```python
from build123d import *

# Parameters (mm, degrees)
F1_DEPTH = 10
F2_W     = 5
F2_H     = 5
F3_DEPTH = 5
F4_W     = 5
F4_H     = 5
F5_DEPTH = 2
F6_SIZE  = 1


with BuildPart() as f1:
    # F0 (on Front) → F1 (new body)
    with BuildSketch(Plane.XZ):
        Polygon((0, 49.2), (0, 0), (21.76041, 48.874682), (14.42041, 48.874682), (6.8, 31.7), (6.8, 49.2), align=None)
    extrude(amount=F1_DEPTH)

    # F2 (on face) → F3 (cut)
    with BuildSketch(Plane.XY.offset(49.2)):
        with Locations((3.4, -5)):
            Rectangle(F2_W, F2_H)
    extrude(amount=-F3_DEPTH, mode=Mode.SUBTRACT)

    # F4 (on face) → F5 (cut)
    with BuildSketch(Plane.XY.offset(48.874682)):
        with Locations((18.09041, -5)):
            Rectangle(F4_W, F4_H)
    extrude(amount=-F5_DEPTH, mode=Mode.SUBTRACT)

    # F6
    f6_edges = [f1.edges().sort_by_distance(p)[0] for p in [
        (6.8, -10, 40.45),
        (0, -10, 24.6),
        (10.610205, -10, 40.287341),
        (6.8, 0, 40.45),
        (10.880205, 0, 24.437341),
        (10.610205, 0, 40.287341),
        (10.880205, -10, 24.437341),
        (0, 0, 24.6),
    ]]
    chamfer(f6_edges, length=F6_SIZE)


solid = f1.part
```
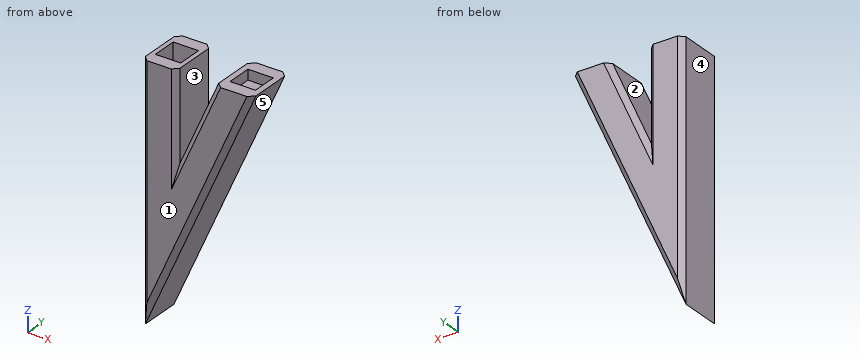
Model file for the job. Use its own axes, mm. Face numbers are marked on the shaded views. A direction names the side the tool comes from. Coordinates: 2 decimals unless noted, no trailing zeros. Write each loop counter-clockwise with the first axis right and the second up, starting at its lowest first coordinate (ties: lowest second). Pieces come first, ordered by that corner, then holes. Notation, with made-up numbers: (-18.5, -18) - (22.5, -18) arc R24 cw to (22.5, -4) - close; hole circle Ø7 at (-3, 33.25). An arc over 180 degrees is marked (long way). Use a Markdown table: item, result. Add a question column.
Item 1: 3-axis set-ups, long thin cutter, end or side, ignore diameter. For the marked faces 1 and 2: which of +Z, -Z, +X, -X, +Y, -Y reach the whole face in a straight line?
Item 2: Band-saw the part on D-D, the plane z = 21.5. Write the cut outline in (x, y).
Item 3: Two-plate mould, pull along X, no slides. Class the marked faces 3, 4 and 5: pulls with the +X half, pulls with the -X half, needs draft (parallel to the pull), parting line crosses it, or undercut.
Item 4: Band-saw the part on B-B, the plane z = 41.5. Write the cut outline in (x, y), and give its area (3 significant figures).
Item 5: Band-saw the part on A-A, the plane y = -4.25. Write the cut outline in (x, z), and give its area (3 significant figures).
Item 6: Drill centre lines: line 1 along X through (y, z) = (-2, 40); line 2 along X through (y, z) = (-9, 37.5); line 3 along Y through (x, z) = (18.75, 44). Where is each one in solid material? Low to high.
Item 7: Band-saw the part on C-C, the plane x = 2.5. Write the cut outline in (y, z), and give its area (3 significant figures).
Item 8: Drop flat-ended pins along their axis: pin 1 (2 mm diameter, centred on y = -1.5, z = 21, fed in from +X); pin 2 (2.5 mm diameter, centred on y = -5, z = 47.5, fed in from +X); pin 3 (6 mm diameter, centred on x = 16.5, y = -8, fed in from +Z); pin 4 (10 mm diameter, centred on x = 7, z = 37.5, fed in from +Y). Give the stop position or say it passes through.
A:
| question | item | result |
|---|---|---|
| 1 | face 1 | +Z, -Z, +X, -X, -Y |
| 1 | face 2 | +Z, +Y, -Y |
| 2 | outline | (0, -9) - (1, -10) - (8.48, -10) - (9.57, -9) - (9.57, -1) - (8.48, 0) - (1, 0) - (0, -1) - close |
| 3 | face 3 | undercut |
| 3 | face 4 | pulls with the -X half |
| 3 | face 5 | pulls with the +X half |
| 4 | outline | (0, -9) - (1, -10) - (5.8, -10) - (6.8, -9) - (6.8, -1) - (5.8, 0) - (1, 0) - (0, -1) - close; (11.15, -9) - (12.24, -10) - (17.38, -10) - (18.48, -9) - (18.48, -1) - (17.38, 0) - (12.24, 0) - (11.15, -1) - close |
| 4 | area | 137 mm² |
| 5 | outline | (0, 0) - (21.76, 48.87) - (20.59, 48.87) - (20.59, 46.87) - (15.59, 46.87) - (15.59, 48.87) - (14.42, 48.87) - (6.8, 31.7) - (6.8, 49.2) - (5.9, 49.2) - (5.9, 44.2) - (0.9, 44.2) - (0.9, 49.2) - (0, 49.2) - close |
| 5 | area | 434 mm² |
| 6 | line 1 | x = 0 to 6.8, 10.48 to 17.81 |
| 6 | line 2 | x = 0 to 6.8, 9.37 to 16.7 |
| 6 | line 3 | y = -9.77 to -0.23 |
| 7 | outline | (-10, 8.07) - (-9, 5.62) - (-1, 5.62) - (0, 8.07) - (0, 49.2) - (-2.5, 49.2) - (-2.5, 44.2) - (-7.5, 44.2) - (-7.5, 49.2) - (-10, 49.2) - close |
| 7 | area | 408 mm² |
| 8 | pin 1 | stops at x = 9.8 |
| 8 | pin 2 | stops at x = 21.7 |
| 8 | pin 3 | stops at z = 48.87 |
| 8 | pin 4 | stops at y = 0 |
